Verification items for the finished model (mm, model axes). Face numbers are marked on the shaded views. A direction names the side the tool comes from. Give positions to 0.01 mm unless a question says otherwise; leave off trailing zeros. Write each loop counter-clockwise with the first axis right and the second up, starting at its lowest first coordinate (ties: lowest second). Pieces come first, ordered by that corner, then holes.
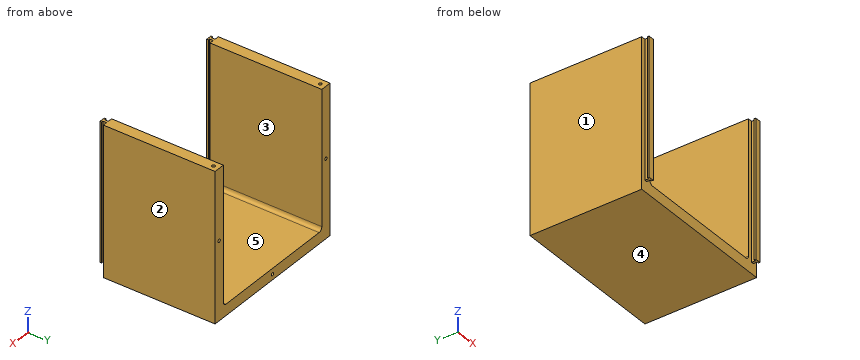
from build123d import *

# Parameters (mm, degrees)
BOSS_EXTRUDE1_DEPTH = 225
BOSS_EXTRUDE2_DEPTH = 10
SKETCH6_W           = 210
SKETCH6_H           = 200
BOSS_EXTRUDE3_DEPTH = 15
SKETCH5_R           = 2.1
CUT_EXTRUDE1_DEPTH  = 4.5
SKETCH10_W          = 210
SKETCH10_H          = 200
BOSS_EXTRUDE4_DEPTH = 40
SKETCH11_R          = 5
BOSS_EXTRUDE5_DEPTH = 5
BOSS_EXTRUDE5_TAPER = 5
SKETCH13_W          = 185
SKETCH13_H          = 10
BOSS_EXTRUDE6_DEPTH = 47.5
SKETCH14_W          = 185
SKETCH14_H          = 10
BOSS_EXTRUDE7_DEPTH = 47.5
SKETCH7_W           = 21
SKETCH7_H           = 10.25
CUT_EXTRUDE2_DEPTH  = 15
SKETCH15_R          = 2.1
CUT_EXTRUDE4_DEPTH  = 6
BOSS_EXTRUDE8_DEPTH = 185
FILLET1_R           = 5


with BuildPart() as part:
    # Sketch2 → Boss-Extrude1 (new body)
    with BuildSketch(Plane(origin=(0, 0, 0), x_dir=(1, 0, 0), z_dir=(0, 1, 0))):
        Polygon((-90, 0), (90, 0), (90, -185), (105, -185), (105, 15), (-105, 15), (-105, -185), (-90, -185), align=None)
    extrude(amount=BOSS_EXTRUDE1_DEPTH)

    # Sketch3 → Boss-Extrude2 (add)
    with BuildSketch(Plane(origin=(0, 10, 0), x_dir=(1, 0, 0), z_dir=(0, 1, 0))):
        Polygon((-90, -185), (-22.5, -185), (-22.5, -10), (22.5, -10), (22.5, -185), (90, -185), (90, 0), (-90, 0), align=None)
    extrude(amount=BOSS_EXTRUDE2_DEPTH)

    # Sketch6 → Boss-Extrude3 (add)
    with BuildSketch(Plane.XZ):
        with Locations((0, 85)):
            Rectangle(SKETCH6_W, SKETCH6_H)
    extrude(amount=BOSS_EXTRUDE3_DEPTH)

    # Sketch5 → Cut-Extrude1 (cut)
    with BuildSketch(Plane.XY.offset(185)):
        with Locations((-97.5, 217.5)):
            Circle(SKETCH5_R)
        with Locations((97.5, 217.5)):
            Circle(SKETCH5_R)
        with Locations((-97.5, -7.5)):
            Circle(SKETCH5_R)
        with Locations((97.5, -7.5)):
            Circle(SKETCH5_R)
    extrude(amount=-CUT_EXTRUDE1_DEPTH, mode=Mode.SUBTRACT)

    # Sketch10 → Boss-Extrude4 (add)
    with BuildSketch(Plane.XZ.offset(15)):
        with Locations((0, 85)):
            Rectangle(SKETCH10_W, SKETCH10_H)
    extrude(amount=BOSS_EXTRUDE4_DEPTH)

    # Sketch11 → Boss-Extrude5 (add)
    with BuildSketch(Plane(origin=(0, 0, 0), x_dir=(1, 0, 0), z_dir=(0, 1, 0))):
        with Locations((0, -90)):
            Circle(SKETCH11_R)
    extrude(amount=BOSS_EXTRUDE5_DEPTH, taper=BOSS_EXTRUDE5_TAPER)

    # Sketch13 → Boss-Extrude6 (add)
    with BuildSketch(Plane.ZY.offset(-90)):
        with Locations((92.5, 5)):
            Rectangle(SKETCH13_W, SKETCH13_H)
    extrude(amount=BOSS_EXTRUDE6_DEPTH)

    # Sketch14 → Boss-Extrude7 (add)
    with BuildSketch(Plane(origin=(-90, 0, 0), x_dir=(0, 0, -1), z_dir=(1, 0, 0))):
        with Locations((-92.5, 5)):
            Rectangle(SKETCH14_W, SKETCH14_H)
    extrude(amount=BOSS_EXTRUDE7_DEPTH)

    # Sketch7 → Cut-Extrude2 (cut)
    with BuildSketch(Plane(origin=(0, 0, -15), x_dir=(-1, 0, 0), z_dir=(0, 0, -1))):
        with Locations((-32, 5.125)):
            Rectangle(SKETCH7_W, SKETCH7_H)
    extrude(amount=-CUT_EXTRUDE2_DEPTH, mode=Mode.SUBTRACT)

    # Sketch15 → Cut-Extrude4 (cut)
    with BuildSketch(Plane(origin=(0, 225, 0), x_dir=(1, 0, 0), z_dir=(0, 1, 0))):
        with Locations((0, 7.5)):
            Circle(SKETCH15_R)
        with Locations((-97.5, -90)):
            Circle(SKETCH15_R)
        with Locations((97.5, -90)):
            Circle(SKETCH15_R)
    extrude(amount=-CUT_EXTRUDE4_DEPTH, mode=Mode.SUBTRACT)

    # Split1
    split(bisect_by=Plane.ZX.offset(75), keep=Keep.TOP)

    # Sketch16 → Boss-Extrude8 (add)
    with BuildSketch(Plane.XY.offset(185)):
        Polygon((-99.15, 75), (-95.85, 75), (-95.85, 70), (-93.65, 70), (-93.65, 67.8), (-101.35, 67.8), (-101.35, 70), (-99.15, 70), align=None)
        Polygon((101.35, 70), (99.15, 70), (99.15, 75), (95.85, 75), (95.85, 70), (93.65, 70), (93.65, 67.8), (101.35, 67.8), align=None)
    extrude(amount=-BOSS_EXTRUDE8_DEPTH)

    # Fillet1
    fillet1_edges = [part.edges().sort_by_distance(p)[0] for p in [
        (90, 150, 0),
        (-90, 150, 0),
    ]]
    fillet(fillet1_edges, radius=FILLET1_R)


solid = part.part
Item 1: Sectioned sample at B-B on y = 190.5. Record the cut outline in (x, z).
Answer key:
outline: (-105, -15) - (105, -15) - (105, 185) - (90, 185) - (90, 5) arc R5 cw to (85, 0) - (-85, 0) arc R5 cw to (-90, 5) - (-90, 185) - (-105, 185) - close
Item 2: Depth check by flat-ended pin: pin 1 (10 mm diameter, centred on x = 15.5, y = 91.5, fed in from +Z); pin 2 (3.5 mm diameter, centred on x = -97.5, z = 90, fed in from +Y); pin 3 (2 mm diameter, centred on x = 97, y = 217, fed in from +Z). Enter the tip coordinate at first touch or a pass-through.
Answer key:
pin 1: stops at z = 0
pin 2: stops at y = 219
pin 3: stops at z = 180.5
Item 3: Release check for a two-part mould opening along X. For the marked faces 1, 2 and 3 record: released by +X, released by -X, zero draft, split by the parting line, or undercut.
Answer key:
face 1: released by -X
face 2: released by +X
face 3: undercut
Item 4: Sectioned sample at A-A on z = 119.5. Record the cut outline in (x, y).
Answer key:
outline: (-105, 75) - (-99.15, 75) - (-99.15, 70) - (-101.35, 70) - (-101.35, 67.8) - (-93.65, 67.8) - (-93.65, 70) - (-95.85, 70) - (-95.85, 75) - (-90, 75) - (-90, 225) - (-105, 225) - close; (90, 75) - (95.85, 75) - (95.85, 70) - (93.65, 70) - (93.65, 67.8) - (101.35, 67.8) - (101.35, 70) - (99.15, 70) - (99.15, 75) - (105, 75) - (105, 225) - (90, 225) - close
Item 5: Scan lines: line 1 along X through (y, z) = (217, 183); line 2 along X through (y, z) = (223, 90); line 3 along X through (y, z) = (221.2, -7.5). Record each from-to range of solid material in increasing order.
Answer key:
line 1: x = -105 to -99.54, -95.46 to -90, 90 to 95.46, 99.54 to 105
line 2: x = -105 to -99.6, -95.4 to -90, 90 to 95.4, 99.6 to 105
line 3: x = -105 to -2.1, 2.1 to 105
Item 6: Set-up check for the marked faces 4 and 5: record each of +Z, -Z, +X, -X, +Y, -Y from which the full face is reachable in a straight line by a thin tool's end or side.
Answer key:
face 4: -Z, +X, -X, +Y, -Y
face 5: +Z, +Y, -Y
Item 7: Sectioned sample at C-C on x = 38.5. Record the cut outline in (y, z).
Answer key:
outline: (75, -15) - (225, -15) - (225, 0) - (75, 0) - close
